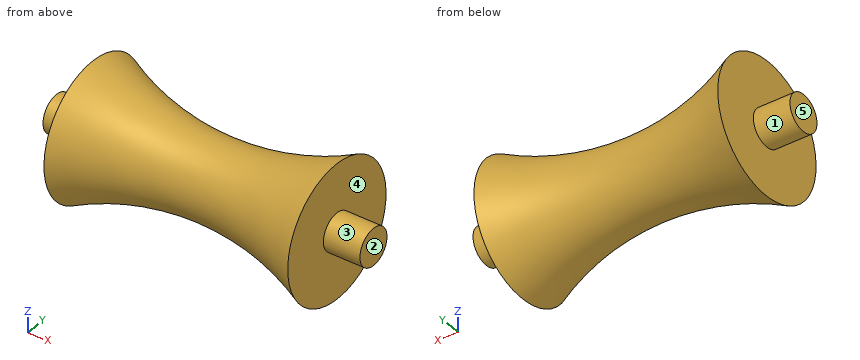
```python
from build123d import *

# Parameters (mm, degrees)
F2_R     = 9.525
F3_DEPTH = 19.05
F4_R     = 9.525
F5_DEPTH = 19.05


with BuildPart() as f1:
    # F0 (on Front) → F1 (revolve)
    with BuildSketch(Plane.XZ):
        with BuildLine():
            ThreePointArc((63.5, 0), (0, -15.24), (-63.5, 0))
            Line((-63.5, 0), (-63.5, -34.633189))
            Line((-63.5, -34.633189), (63.5, -34.633189))
            Line((63.5, -34.633189), (63.5, 0))
        make_face()
    revolve(axis=Axis((0, 0, -34.633189), (-1, 0, 0)))

    # F2 (on face) → F3 (join)
    with BuildSketch(Plane(origin=(-63.5, 0, 0), x_dir=(0, -1, 0), z_dir=(-1, 0, 0))):
        with Locations((0, -34.633189)):
            Circle(F2_R)
    extrude(amount=F3_DEPTH)

    # F4 (on face) → F5 (join)
    with BuildSketch(Plane.YZ.offset(63.5)):
        with Locations((0, -34.633189)):
            Circle(F4_R)
    extrude(amount=F5_DEPTH)


solid = f1.part
```
The listing builds one solid part. Answer for the finished solid, in the listing's coordinates (mm). Face numbers are marked on the shaded views. A direction names the side the tool comes from. Coordinates: 2 decimals unless noted, no trailing zeros. Write each loop counter-clockwise with the first axis right and the second up, starting at its lowest first coordinate (ties: lowest second). Pieces come first, ordered by that corner, then holes. Notation, with made-up numbers: (-27, -35.75) -> (-16, -35.75) arc R25 cw to (-16, -16.75) -> close; hole circle Ø5 at (-38.75, -25.5). An arc over 180 degrees is marked (long way). Write each question's results on one line, items separated by ' | '. Start each with the question number.
1) Flat-ended cylindrical pins translate along their axes: pin 1 Ø1.5 at (y, z) = (-2.5, -51) entering from +X; pin 2 Ø3 at (x, z) = (-3.5, -41) entering from +Y; pin 3 Ø2 at (x, y) = (-10.5, 9) entering from +Z. Find the tip coordinate at first contact, or state that the pin passes through.
2) A tool of negligible diameter and unlimited length cuts with its end or side. For the marked faces 1 and 2, from which of +Z, -Z, +X, -X, +Y, -Y can it reach the whole face along a straight path? Write none if from no direction.
3) For a pull along X with two mould halves and no side action, classify the marked faces 3, 4 and 5 as +X half, -X half, draft (parallel to the pull), parting line (faces both ways), or undercut.
4) A cutting plane is placed at B-B (x = 70.5). Determine the outline of the cut face in (y, z) (3 decimals).
5) Straight lines are drawn through the part: probe 1 along X at (y, z) = (-10, -46); probe 2 along X at (y, z) = (-13, -4); probe 3 along X at (y, z) = (-26.5, -15.5). For each, find the intervals that lie inside material, in ascending order.
6) A cutting plane is placed at A-A (y = 0). Determine the outline of the cut face in (x, z).
Values follow:
1) pin 1: x = 63.5 | pin 2: y = 18.82 | pin 3: z = -16.53
2) face 1: -X | face 2: +Z, -Z, +X, +Y, -Y
3) face 3: draft | face 4: +X half | face 5: -X half
4) outline: circle Ø19.05 at (0, -34.633)
5) probe 1: -63.5 to 63.5 | probe 2: -63.5 to -60.76, 60.76 to 63.5 | probe 3: -63.5 to -59.52, 59.52 to 63.5
6) outline: (-82.55, -44.16) -> (-63.5, -44.16) -> (-63.5, -69.27) arc R139.91 cw to (63.5, -69.27) -> (63.5, -44.16) -> (82.55, -44.16) -> (82.55, -25.11) -> (63.5, -25.11) -> (63.5, 0) arc R139.91 cw to (-63.5, 0) -> (-63.5, -25.11) -> (-82.55, -25.11) -> close
